```python
from build123d import *

# Parameters (mm, degrees)
SKETCH1_W               = 185
SKETCH1_H               = 30
SKETCH1_W_2             = 30
SKETCH1_H_2             = 185
BOSS_EXTRUDE1_DEPTH     = 5
SKETCH2_W               = 5
SKETCH2_H               = 30
BOSS_EXTRUDE2_DEPTH     = 30
CUT_EXTRUDE1_DEPTH      = 299.83105595
CUT_EXTRUDE1_DEPTH_BACK = 299.83105595
SKETCH3_R               = 3
SKETCH4_R               = 3.5
CUT_EXTRUDE2_DEPTH      = 5
FILLET1_R               = 4
FILLET2_R               = 3
FILLET3_R               = 3


with BuildPart() as part:
    # Sketch1 → Boss-Extrude1 (new body)
    with BuildSketch(Plane.XY):
        with Locations((107.5, 0)):
            Rectangle(SKETCH1_W, SKETCH1_H)
        with Locations((0, 107.5)):
            Rectangle(SKETCH1_W_2, SKETCH1_H_2)
        with Locations((-107.5, 0)):
            Rectangle(SKETCH1_W, SKETCH1_H)
        Rectangle(SKETCH1_W_2, SKETCH1_H)
        with Locations((0, -107.5)):
            Rectangle(SKETCH1_W_2, SKETCH1_H_2)
    extrude(amount=BOSS_EXTRUDE1_DEPTH)

    # Sketch2 → Boss-Extrude2 (add)
    with BuildSketch(Plane(origin=(0, 0, 0), x_dir=(-1, 0, 0), z_dir=(0, 0, -1))):
        with Locations((-17.5, 0)):
            Rectangle(SKETCH2_W, SKETCH2_H)
        with Locations((17.5, 0)):
            Rectangle(SKETCH2_W, SKETCH2_H)
    extrude(amount=BOSS_EXTRUDE2_DEPTH)

    # Sketch3 → Cut-Extrude1 (cut, two sides: drawn at the far end of the back side and taken through both)
    with BuildSketch(Plane(origin=(20, 0, 0), x_dir=(0, 0, -1), z_dir=(1, 0, 0)).offset(-CUT_EXTRUDE1_DEPTH_BACK)):
        with Locations((15, 0)):
            Circle(SKETCH3_R)
    extrude(amount=CUT_EXTRUDE1_DEPTH + CUT_EXTRUDE1_DEPTH_BACK, mode=Mode.SUBTRACT)

    # Sketch4 → Cut-Extrude2 (cut)
    with BuildSketch(Plane.XY.offset(5)):
        with Locations((0, 175)):
            Circle(SKETCH4_R)
        with Locations((175, 0)):
            Circle(SKETCH4_R)
        with Locations((0, -175)):
            Circle(SKETCH4_R)
        with Locations((-175, 0)):
            Circle(SKETCH4_R)
    extrude(amount=-CUT_EXTRUDE2_DEPTH, mode=Mode.SUBTRACT)

    # Fillet1
    fillet1_edges = [part.edges().sort_by_distance(p)[0] for p in [
        (200, -15, 2.5),
        (15, -15, 2.5),
        (15, -200, 2.5),
        (-15, -200, 2.5),
        (-15, -15, 2.5),
        (-200, -15, 2.5),
        (-200, 15, 2.5),
        (-15, 15, 2.5),
        (-15, 200, 2.5),
        (15, 200, 2.5),
        (15, 15, 2.5),
        (200, 15, 2.5),
    ]]
    fillet(fillet1_edges, radius=FILLET1_R)

    # Fillet2
    fillet2_edges = [part.edges().sort_by_distance(p)[0] for p in [
        (17, -15, 0),
        (17, 15, 0),
        (17.5, 15, -30),
        (17.5, -15, -30),
    ]]
    fillet(fillet2_edges, radius=FILLET2_R)

    # Fillet3
    fillet3_edges = [part.edges().sort_by_distance(p)[0] for p in [
        (-17, -15, 0),
        (-17, 15, 0),
        (-17.5, -15, -30),
        (-17.5, 15, -30),
    ]]
    fillet(fillet3_edges, radius=FILLET3_R)


solid = part.part
```
Geometry: final body of the model. Coordinates: model frame, mm. A direction names the side the tool comes from. Coordinates: 2 decimals unless noted, no trailing zeros. Order: outer loops, then holes, each group sorted by start corner. A loop starts at its lowest first (then second) coordinate and runs counter-clockwise, first axis right, second up.
Item 1: Draft query along X for faces 4 (the face through (-15, 0, -11)), 5 (the face through (-1, -14, 5)), 6 (the face through (20, -4, -15)). Return one class per face: released by +X, released by -X, zero draft, split by the parting line, or undercut.
Answer:
face 4: undercut
face 5: zero draft
face 6: released by +X
Item 2: Contact query for flat-ended pins moving along their axis: P1, Ø5.5, axis at y = -126, z = 2.5, coming from the -X side; P2, Ø9, axis at x = 139, y = -7, coming from the -Z side; P3, Ø12, axis at y = 156, z = 0.5, coming from the +X side; P4, Ø8, axis at x = 175, y = 0, coming from the +Z side. Output: stop coordinate, or through.
Answer:
P1: stops at x = -15
P2: stops at z = 0
P3: stops at x = 15
P4: stops at z = 5
Item 3: Access query for faces 1 (the face through (-20, -4, -15)), 2 (the face through (109, 0, 0)), 3 (the face through (15, 0, -11)). Directions: +Z, -Z, +X, -X, +Y, -Y. A direction counts if a zero-diameter tool reaches every point of the face in a straight line with its end or side. Return the directions, or none.
Answer:
face 1: -Z, -X, +Y, -Y
face 2: -Z, +X, +Y, -Y
face 3: -Z, +Y, -Y
Item 4: Section query A-A (y = 90.5). Output: boundary loops of the cut face in (x, z), then the cut area to 3 significant figures.
Answer:
outline: (-15, 0) - (15, 0) - (15, 5) - (-15, 5) - close
area: 150 mm2
Item 5: Material intervals for line 1 along Y through (x, z) = (-175, 3.2); line 2 along Y through (x, z) = (0, 2); line 3 along Y through (x, z) = (16.9, -15), sorted ascending.
Answer:
line 1: y = -15 to -3.5, 3.5 to 15
line 2: y = -200 to -178.5, -171.5 to 171.5, 178.5 to 200
line 3: y = -15 to -3, 3 to 15
